Can you work these out from the model? Positions are in its coordinate system, mm. Face numbers are marked on the shaded views. A direction names the side the tool comes from. Coordinates: 2 decimals unless noted, no trailing zeros. Loops run counter-clockwise (first coordinate to the right, second up) from the corner with the lowest first, then second, coordinate; pieces in that order, holes last. Notation, with made-up numbers: M -26.5,71 L 20.5,71 A21 cw 20.5,106 Z; hole C 10.5,-16 d7. An arc over 180 degrees is marked long. Answer as a JSON object with one key per item and string values. Group by question number.
Item 1: I'm going to push flat-ended pins straight in: pin 1 Ø3 at (y, z) = (-15.5, -24.5) entering from +X; pin 2 Ø5 at (y, z) = (-11.5, -12) entering from +X; pin 3 Ø3 at (x, z) = (28.5, -51.5) entering from -Y; pin 4 Ø1 at (x, z) = (95.5, 54.5) entering from -Y. Where does each tip first touch, or does it pass through?
Item 2: Suppose I cut it at A-A (x = -82.5). Write out the boundary of the cut face in (y, z), then the cut area to 3 significant figures.
Item 3: We'd pull the mould along Z, two halves only. Please class the marked faces 3, 4 and 5: +Z half, -Z half, draft (parallel to the pull), parting line (faces both ways), or undercut.
Item 4: Suppose I cut it at B-B (y = -8). Write out the boundary of the cut face in (x, z).
Item 5: If I drill on line 1 (X direction, y = -7.5, z = -3); line 2 (Z direction, x = 58, y = -11.25); line 3 (Z direction, x = 110.5, y = 1.25), over which ranges is the centre line in solid material (lowest first)?
Item 6: Which directions (+Z, -Z, +X, -X, +Y, -Y) give clear straight access to the entire face, cutting with the end or side of a thin tool? Please do the marked faces 1 and 2.
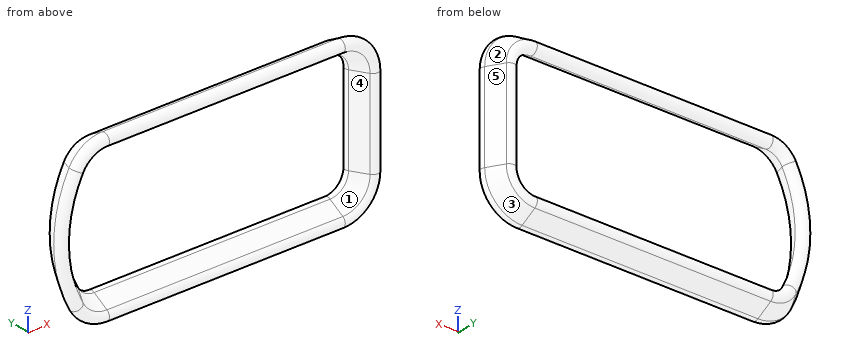
```python
from build123d import *


with BuildPart() as part:
    # Austragung2: sweep along a path in Skizze1
    with BuildLine(Plane(origin=(0, 0, 0), x_dir=(1, 0, 0), z_dir=(0, 1, 0))) as austragung2_path:
        Line((-100.35104183, -57.432811357), (100.35104183, -57.432811357))
        ThreePointArc((100.35104183, -57.432811357), (114.493177454, -51.574946981), (120.35104183, -37.432811357))
        Line((120.35104183, -37.432811357), (120.35104183, 37.432811357))
        ThreePointArc((120.35104183, 37.432811357), (114.493177454, 51.574946981), (100.35104183, 57.432811357))
        Line((100.35104183, 57.432811357), (-100.35104183, 57.432811357))
        ThreePointArc((-100.35104183, 57.432811357), (-110.666950496, 54.567046922), (-118.026562745, 46.791014197))
        ThreePointArc((-118.026562745, 46.791014197), (-129.64895817, 0), (-118.026562745, -46.791014197))
        ThreePointArc((-118.026562745, -46.791014197), (-110.666950496, -54.567046922), (-100.35104183, -57.432811357))
    # Skizze2 → Austragung2 (sweep)
    with BuildSketch(Plane.XY):
        with BuildLine():
            Line((-125.318831151, -2.5), (-132.818831151, -15.490381057))
            ThreePointArc((-132.818831151, -15.490381057), (-139.64895817, -17.320508076), (-141.479085189, -10.490381057))
            Line((-141.479085189, -10.490381057), (-133.979085189, 2.5))
            ThreePointArc((-133.979085189, 2.5), (-127.14895817, 4.330127019), (-125.318831151, -2.5))
        make_face()
    sweep(path=austragung2_path.line)


solid = part.part
```
From the geometry:
{
 "1": {"pin 1": "x = 132.75", "pin 2": "x = 132.85", "pin 3": "y = -2.31", "pin 4": "y = -5.79"},
 "2": {"outline": "M -15.49,-60.6 A5 ccw -10.49,-69.26 L 2.5,-61.76 A5 ccw -2.5,-53.1 Z; M -15.49,60.6 L -2.5,53.1 A5 ccw 2.5,61.76 L -10.49,69.26 A5 ccw Z", "area": "457 mm2"},
 "3": {"face 3": "-Z half", "face 4": "undercut", "face 5": "draft"},
 "4": {"outline": "M -127.21,-51.65 A30.39 ccw -100.35,-67.83 L 100.35,-67.83 A30.39 ccw 130.74,-37.43 L 130.74,37.43 A30.39 ccw 100.35,67.83 L -100.35,67.83 A30.39 ccw -127.21,51.65 A110.39 ccw Z; hole M -117.01,-46.25 A18.85 ccw -100.35,-56.28 L 100.35,-56.28 A18.85 ccw 119.2,-37.43 L 119.2,37.43 A18.85 ccw 100.35,56.28 L -100.35,56.28 A18.85 ccw -117.01,46.25 A98.85 ccw Z"},
 "5": {"line 1": "-139.71 to -128.16, 118.91 to 130.45", "line 2": "-69.62 to -58.15, 58.15 to 69.62", "line 3": "-60.34 to -48.69, 48.69 to 60.34"},
 "6": {"face 1": "-Y", "face 2": "+Z, +X, +Y"}
}
